Input: part model. Units: mm. Frame: model coordinates. Face numbers are marked on the shaded views. A direction names the side the tool comes from. Round coordinates to 2 decimals unless told otherwise and drop trailing zeros. Loops run counter-clockwise (first coordinate to the right, second up) from the corner with the lowest first, then second, coordinate; pieces in that order, holes last.
1) Draft query along X for the marked faces 4, 5 and 6. Return one class per face: pulls with the +X half, pulls with the -X half, needs draft (parallel to the pull), parting line crosses it, or undercut.
2) First-contact query: pin 1 (21 mm diameter, centred on y = 26.5, z = -4, fed in from -X); pin 2 (9.5 mm diameter, centred on x = 4, z = 3, fed in from +Y); pin 3 (20.5 mm diameter, centred on x = -0.5, z = -1, fed in from +Y); pin 4 (11.5 mm diameter, centred on x = 0, z = 0, fed in from -Y). Flat tips, straight axial feed; report the tip coordinate or a pass-through.
3) Ray query, line 1 along X through (y, z) = (8, 0); line 2 along Y through (x, z) = (16, 0); line 3 along X through (y, z) = (23, 8.5). Return the intervals inside material, ascending.
4) Section A-A, the plane z = 0. Return loops of the section in (x, y).
5) Section C-C, the plane y = 15.5. Return loops of the section in (x, z), and give its area (3 significant figures).
6) Section D-D, the plane y = 31.5. Return loops of the section in (x, z).
7) Access query for the marked faces 1, 2 and 3. Directions: +Z, -Z, +X, -X, +Y, -Y. A direction counts if a zero-diameter tool reaches every point of the face in a straight line with its end or side. Return the directions, or none.
8) Section B-B, the plane x = 0. Return loops of the section in (y, z).
from build123d import *

# Parameters (mm, degrees)
SKETCH_1_W               = 42.2
SKETCH_1_H               = 45
EXTRUDE_1_DEPTH          = 9.5
EXTRUDE_2_DEPTH          = 36.7
SKETCH_4_W               = 25.7
SKETCH_4_H               = 42.5
CUT_EXTRUDE_1_DEPTH      = 23.5
CUT_EXTRUDE_1_DEPTH_BACK = 23.5
CHAMFER_1_SIZE           = 2
HOLE_WIZARD_M81_2_D      = 6.8
HOLE_WIZARD_M81_2_DEPTH  = 5.5


with BuildPart() as part:
    # Эскиз1 → Бобышка-Вытянуть1 (new body)
    with BuildSketch(Plane(origin=(0, 0, 0), x_dir=(1, 0, 0), z_dir=(0, 1, 0))):
        Rectangle(SKETCH_1_W, SKETCH_1_H)
    extrude(amount=EXTRUDE_1_DEPTH)

    # Эскиз2 → Вырез-Повернуть1 (revolve, cut)
    with BuildSketch(Plane.XY):
        Polygon((-6.25, 0), (-6.25, 4.75), (-9.5, 4.75), (-9.5, 9.5), (0, 9.5), (0, 0), align=None)
    revolve(axis=Axis((0, 9.5, 0), (0, -1, 0)), mode=Mode.SUBTRACT)

    # Эскиз3 → Бобышка-Вытянуть2 (add)
    with BuildSketch(Plane(origin=(21.1, 0, 0), x_dir=(0, 0, -1), z_dir=(1, 0, 0))):
        with BuildLine():
            Line((-22.5, 9.5), (-20.422219056, 33.284087671))
            ThreePointArc((-20.422219056, 33.284087671), (0, 52), (20.422219056, 33.284087671))
            Line((20.422219056, 33.284087671), (22.5, 9.5))
            Line((22.5, 9.5), (-22.5, 9.5))
        make_face()
    extrude(amount=-EXTRUDE_2_DEPTH)

    # Эскиз4 → Вырез-Вытянуть1 (cut, two sides)
    with BuildSketch(Plane.XY) as cut_extrude_1_sk:
        with Locations((2.75, 30.75)):
            Rectangle(SKETCH_4_W, SKETCH_4_H)
    extrude(amount=CUT_EXTRUDE_1_DEPTH, mode=Mode.SUBTRACT)
    extrude(cut_extrude_1_sk.sketch, amount=-CUT_EXTRUDE_1_DEPTH_BACK, mode=Mode.SUBTRACT)

    # Фаска1
    chamfer_1_edges = [part.edges().sort_by_distance(p)[0] for p in [
        (-21.1, 4.75, -22.5),
        (-21.1, 4.75, 22.5),
    ]]
    chamfer(chamfer_1_edges, length=CHAMFER_1_SIZE)

    # Эскиз10 → Hole Wizard M81 (revolve, cut)
    with BuildSketch(Plane(origin=(21.1, 31.5, 0), x_dir=(0, 0, -1), z_dir=(0, 1, 0))):
        Polygon((0, 0), (0, 5.5), (4.25, 5.5), (4.25, 4.25), (8.5, 0), align=None)
    revolve(axis=Axis((27.45, 31.5, 0), (-1, 0, 0)), mode=Mode.SUBTRACT)

    # Hole Wizard M81 2
    with Locations(Plane.ZY.offset(15.6)):
        with Locations((0, 31.5)):
            Hole(HOLE_WIZARD_M81_2_D / 2, depth=HOLE_WIZARD_M81_2_DEPTH)


solid = part.part
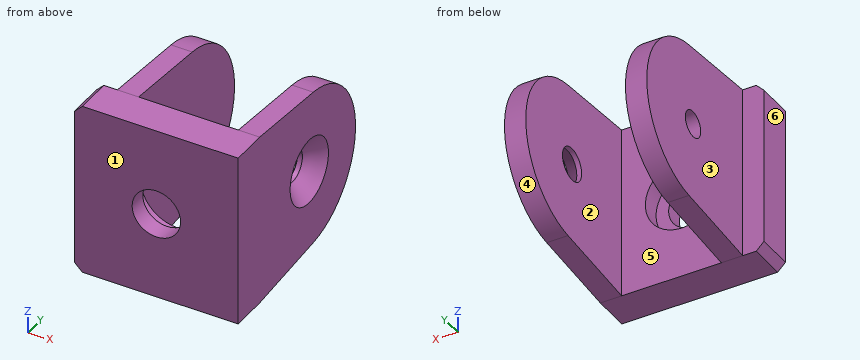
Final values:
1. face 4: needs draft
1. face 5: undercut
1. face 6: pulls with the -X half
2. pin 1: stops at x = -15.6
2. pin 2: stops at y = 9.5
2. pin 3: stops at y = 52
2. pin 4: passes through
3. line 1: x = -21.1 to -9.5, 9.5 to 21.1
3. line 2: y = 0 to 27.25, 35.75 to 52
3. line 3: x = -15.6 to -10.1, 15.6 to 21.1
4. outline: (-21.1, 0) - (-6.25, 0) - (-6.25, 4.75) - (-9.5, 4.75) - (-9.5, 9.5) - (-10.1, 9.5) - (-10.1, 28.1) - (-15.6, 28.1) - (-15.6, 9.5) - (-21.1, 9.5) - close; (-15.6, 34.9) - (-10.1, 34.9) - (-10.1, 52) - (-15.6, 52) - close; (6.25, 0) - (21.1, 0) - (21.1, 23) - (16.85, 27.25) - (15.6, 27.25) - (15.6, 9.5) - (9.5, 9.5) - (9.5, 4.75) - (6.25, 4.75) - close; (15.6, 35.75) - (16.85, 35.75) - (21.1, 40) - (21.1, 52) - (15.6, 52) - close
5. outline: (-15.6, -21.98) - (-10.1, -21.98) - (-10.1, 21.98) - (-15.6, 21.98) - close; (15.6, -21.98) - (21.1, -21.98) - (21.1, 21.98) - (15.6, 21.98) - close
5. area: 483 mm2
6. outline: (-15.6, -20.58) - (-10.1, -20.58) - (-10.1, -3.4) - (-15.6, -3.4) - close; (-15.6, 3.4) - (-10.1, 3.4) - (-10.1, 20.58) - (-15.6, 20.58) - close; (15.6, -20.58) - (21.1, -20.58) - (21.1, -8.5) - (16.85, -4.25) - (15.6, -4.25) - close; (15.6, 4.25) - (16.85, 4.25) - (21.1, 8.5) - (21.1, 20.58) - (15.6, 20.58) - close
7. face 1: +Z, -Z, +X, -X, -Y
7. face 2: +Z, -Z, +Y
7. face 3: +Z, -Z, -X, +Y
8. outline: (0, -22.5) - (9.5, -22.5) - (9.5, -9.5) - (4.75, -9.5) - (4.75, -6.25) - (0, -6.25) - close; (0, 6.25) - (4.75, 6.25) - (4.75, 9.5) - (9.5, 9.5) - (9.5, 22.5) - (0, 22.5) - close
